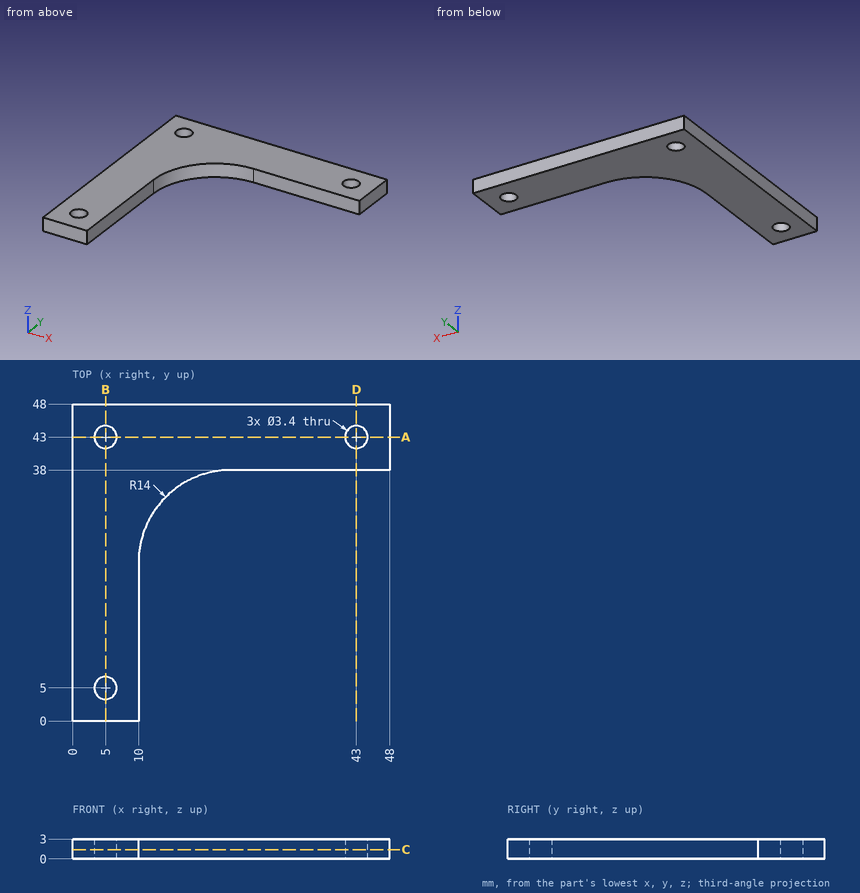
Print and shaded views of the part. All mm, measured from the part's lowest x, y and z. Coordinates: 2 decimals unless noted, no trailing zeros. Loops run counter-clockwise (first coordinate to the right, second up) from the corner with the lowest first, then second, coordinate; pieces in that order, holes last. Notation, with made-up numbers: (8.5, -34.75) - (20.5, -34.75) arc R19 cw to (20.5, -4.75) - close; hole circle Ø11 at (62.25, -27). An arc over 180 degrees is marked (long way). Write item = value, one per line. Start each with the question number.
Item 1: Flat gauge pins, fed straight in: pin 1 Ø3 at (x, y) = (43, 43) entering from -Z; pin 2 Ø1 at (x, z) = (30, 0.5) entering from -Y; pin 3 Ø1.5 at (y, z) = (13, 2) entering from +X. Where does each tip first touch, or does it go through?
Item 2: Wall check: L1, parallel to Y at x = 5, z = 0.7; L2, parallel to Y at x = 6, z = 1.55; L3, parallel to Y at x = 43, z = 2. Give the ranges that are in metal, low to high. Write a range as from..to.
Item 3: Cut at D-D, the plane x = 43. Give the cut face in (y, z).
Item 4: Cut at A-A, the plane y = 43. Give the cut face in (x, z).
Item 5: Cut at C-C, the plane z = 1.4. Give the cut face in (x, y).
The answers:
q1.pin_1 = through
q1.pin_2 = 38
q1.pin_3 = 10
q2.L1 = 0..3.3, 6.7..41.3, 44.7..48
q2.L2 = 0..3.63, 6.37..41.63, 44.37..48
q2.L3 = 38..41.3, 44.7..48
q3.outline = (38, 0) - (41.3, 0) - (41.3, 3) - (38, 3) - close; (44.7, 0) - (48, 0) - (48, 3) - (44.7, 3) - close
q4.outline = (0, 0) - (3.3, 0) - (3.3, 3) - (0, 3) - close; (6.7, 0) - (41.3, 0) - (41.3, 3) - (6.7, 3) - close; (44.7, 0) - (48, 0) - (48, 3) - (44.7, 3) - close
q5.outline = (0, 0) - (10, 0) - (10, 24) arc R14 cw to (24, 38) - (48, 38) - (48, 48) - (0, 48) - close; hole circle Ø3.4 at (5, 5); hole circle Ø3.4 at (5, 43); hole circle Ø3.4 at (43, 43)
